Source: CAD feature listing. Evaluate the final solid. Frame: model axes, mm. Face numbers are marked on the shaded views. A direction names the side the tool comes from. Give positions to 0.01 mm unless a question says otherwise; leave off trailing zeros. Order: outer loops, then holes, each group sorted by start corner. A loop starts at its lowest first (then second) coordinate and runs counter-clockwise, first axis right, second up. Notation, with made-up numbers: (7.25, 68) - (21.25, 68) arc R11 ccw to (21.25, 88) - close; hole circle Ø9 at (-7, 29). An arc over 180 degrees is marked (long way). Answer as CSV lines item,"result".
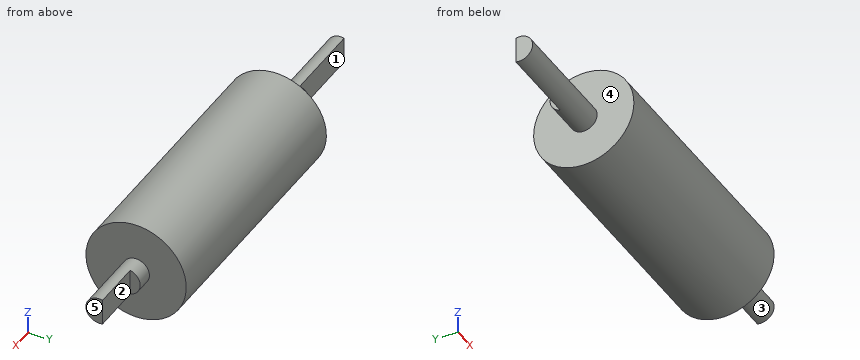
```python
from build123d import *

# Parameters (mm, degrees)
ESBO_O8_R                = 4
RESSALTO_EXTRUS_O4_DEPTH = 35
ESBO_O9_R                = 15
RESSALTO_EXTRUS_O5_DEPTH = 76
ESBO_O10_R               = 4
RESSALTO_EXTRUS_O6_DEPTH = 20
ESBO_O11_W               = 11.087956956
ESBO_O11_H               = 3
CORTE_EXTRUS_O1_DEPTH    = 24
ESBO_O12_W               = 18.763421195
ESBO_O12_H               = 3
CORTE_EXTRUS_O2_DEPTH    = 15


with BuildPart() as part:
    # Esboço8 → Ressalto-extrusão4 (new body)
    with BuildSketch(Plane(origin=(0, 0, 0), x_dir=(0, 0, -1), z_dir=(1, 0, 0))):
        Circle(ESBO_O8_R)
    extrude(amount=RESSALTO_EXTRUS_O4_DEPTH)

    # Esboço9 → Ressalto-extrusão5 (add)
    with BuildSketch(Plane(origin=(35, 0, 0), x_dir=(0, 0, -1), z_dir=(1, 0, 0))):
        Circle(ESBO_O9_R)
    extrude(amount=RESSALTO_EXTRUS_O5_DEPTH)

    # Esboço10 → Ressalto-extrusão6 (add)
    with BuildSketch(Plane(origin=(111, 0, 0), x_dir=(0, 0, -1), z_dir=(1, 0, 0))):
        Circle(ESBO_O10_R)
    extrude(amount=RESSALTO_EXTRUS_O6_DEPTH)

    # Esboço11 → Corte-extrusão1 (cut)
    with BuildSketch(Plane.ZY):
        with Locations((0, 2.5)):
            Rectangle(ESBO_O11_W, ESBO_O11_H)
    extrude(amount=-CORTE_EXTRUS_O1_DEPTH, mode=Mode.SUBTRACT)

    # Esboço12 → Corte-extrusão2 (cut)
    with BuildSketch(Plane(origin=(131, 0, 0), x_dir=(0, 0, -1), z_dir=(1, 0, 0))):
        with Locations((-0.1910881, 2.5)):
            Rectangle(ESBO_O12_W, ESBO_O12_H)
    extrude(amount=-CORTE_EXTRUS_O2_DEPTH, mode=Mode.SUBTRACT)


solid = part.part
```
(1) Cut plane B-B (y = -7.25). Return loops of the section in (x, z), then the cut area to 3 significant figures.
Completed:
outline,"(35, -13.13) - (111, -13.13) - (111, 13.13) - (35, 13.13) - close"
area,"2,000 mm²"
(2) Cut plane C-C (z = 13). Return loops of the section in (x, y), then the cut area to 3 significant figures.
Completed:
outline,"(35, -7.48) - (111, -7.48) - (111, 7.48) - (35, 7.48) - close"
area,"1,140 mm²"
(3) Access query for the marked faces 1, 2, 3, 4 and 5. Directions: +Z, -Z, +X, -X, +Y, -Y. A direction counts if a zero-diameter tool reaches every point of the face in a straight line with its end or side. Return the directions, or none.
Completed:
face 1,"+Z, -Z, -X, +Y"
face 2,"+Z, -Z, +X, +Y"
face 3,"+X"
face 4,"-X"
face 5,"+Z, -Z, +X, +Y, -Y"
(4) Contact query for flat-ended pins moving along their axis: pin 1 (6 mm diameter, centred on x = 17, z = 0, fed in from +Y); pin 2 (2 mm diameter, centred on x = 41, y = -5, fed in from -Z); pin 3 (6 mm diameter, centred on x = 116.5, y = -1.5, fed in from -Z). Output: stop coordinate, or through.
Completed:
pin 1,"y = 1"
pin 2,"z = -14.46"
pin 3,"z = -4"
(5) Ray query, line 1 (X direction, y = 2.75, z = 1.75); line 2 (X direction, y = -0.5, z = -5); line 3 (Z direction, x = 114, y = 0). Return the intervals inside material, ascending. Write a range as from..to.
Completed:
line 1,"24..116"
line 2,"35..111"
line 3,"-4..4"
(6) Cut plane A-A (z = 0). Return loops of the section in (x, y).
Completed:
outline,"(0, -4) - (35, -4) - (35, -15) - (111, -15) - (111, -4) - (131, -4) - (131, 1) - (116, 1) - (116, 4) - (111, 4) - (111, 15) - (35, 15) - (35, 4) - (24, 4) - (24, 1) - (0, 1) - close"
